Can you work these out from the model? Positions are in its coordinate system, mm. A direction names the side the tool comes from. Give positions to 0.01 mm unless a question says otherwise; leave off trailing zeros. Loops run counter-clockwise (first coordinate to the right, second up) from the corner with the lowest first, then second, coordinate; pieces in that order, holes last. Notation, with made-up numbers: (31, 59) - (74, 59) arc R22 cw to (74, 87) - close; hole circle Ø9 at (12, 85.25). An arc over 180 degrees is marked (long way). Answer as a JSON object with one key per item and string values. Group by question number.
Item 1: Thinking about a two-plate mould opening in X: for faces 3 (the flat face through (0, -2, 3)), 4 (the cylindrical face through (6.302, -1.973, 4.177)), 5 (the flat face through (3.8, 0, 3.1)), 6 (the flat face through (10, -2, 1)), which applies, pulls with the +X half, pulls with the -X half, needs draft (parallel to the pull), parting line crosses it, or undercut?
Item 2: Suppose I cut it at A-A on z = 1.25. Write out the boundary of the cut face in (x, y).
Item 3: Will this pin go through, and if not, where does the flat tip stop? pin 1 (1 mm diameter, centred on x = 5.5, y = -0.5, fed in from -Z).
Item 4: Which directions (+Z, -Z, +X, -X, +Y, -Y) give clear straight access to the entire face, cutting with the end or side of a thin tool? Please do faces 1 (the flat face through (9, -2, 1)), 2 (the flat face through (9.4, -2, 0)).
Item 5: Please list where these lines run through material, in increasing order: L1, parallel to Y at x = 2, z = 2.7; L2, parallel to X at y = -3.75, z = 2.8; L3, parallel to X at y = -3.55, z = 3.3.
Item 6: Suppose I cut it at B-B on x = 2. Write out the boundary of the cut face in (y, z), and give its area (3 significant figures).
from build123d import *

# Parameters (mm, degrees)
F1_DEPTH = 4
F3_R     = 0.1
F2_R     = 0.75
F4_DEPTH = 25


# Not quite as in the source:
# - ends of sketch curves that miss each other by under 0.0002 mm in the source are joined


with BuildPart() as f1:
    # F0 (on Front) → F1 (new body)
    with BuildSketch(Plane.XZ):
        with BuildLine():
            Line((0, 5), (0, 0))
            Line((0, 0), (3.7373243831, 0))
            Line((3.7373243831, 0), (3.7373243831, 1.5373318456))
            ThreePointArc((3.7373243831, 1.5373318456), (6.3598005329, 4.1775164411), (8.9999850781, 1.5550552132))
            Line((8.9999850781, 1.5550552132), (9, 1.5461935545))
            Line((9, 1.5461935545), (9, 0))
            Line((9, 0), (9.6543736474, 0))
            ThreePointArc((9.6543736474, 0), (9.9125401886, 0.7540174245), (10, 1.5461935545))
            ThreePointArc((10, 1.5461935545), (9.3062869056, 3.680900869), (7.4901947663, 5))
            Line((7.4901947663, 5), (5.2471296168, 5))
            Line((5.2471296168, 5), (0, 5))
        make_face()
        with BuildLine():
            Line((10, 0), (10, 1.5461935545))
            ThreePointArc((10, 1.5461935545), (9.9125401886, 0.7540174245), (9.6543736474, 0))
            Line((9.6543736474, 0), (10, 0))
        make_face()
    extrude(amount=F1_DEPTH)

    # F3
    f3_edges = [f1.edges().sort_by_distance(p)[0] for p in [
        (3.745097, -4, 5),
        (0, -2, 5),
        (0, -4, 2.5),
        (6.359793, -4, 4.177516),
        (3.737324, -2, 0),
        (1.868662, -4, 0),
        (9.5, -4, 0),
        (10, -2, 0),
        (9.5, 0, 0),
        (10, 0, 0.773097),
        (10, -4, 0.773097),
        (3.737324, 0, 0.768666),
        (3.745097, 0, 5),
        (0, 0, 2.5),
        (1.868662, 0, 0),
        (0, -2, 0),
    ]]
    fillet(f3_edges, radius=F3_R)

    # F2 (on face) → F4 (cut)
    with BuildSketch(Plane.XY.offset(5)):
        with Locations((2, -2)):
            Circle(F2_R)
    extrude(amount=-F4_DEPTH, mode=Mode.SUBTRACT)


solid = f1.part
Worked out:
{
 "1": {"face 3": "pulls with the -X half", "face 4": "undercut", "face 5": "needs draft", "face 6": "pulls with the +X half"},
 "2": {"outline": "(0, -3.9) arc R0.1 ccw to (0.1, -4) - (3.64, -4) arc R0.1 ccw to (3.74, -3.9) - (3.74, -0.1) arc R0.1 ccw to (3.64, 0) - (0.1, 0) arc R0.1 ccw to (0, -0.1) - close; (9, -3.9) arc R0.1 ccw to (9.1, -4) - (9.9, -4) arc R0.1 ccw to (10, -3.9) - (10, -0.1) arc R0.1 ccw to (9.9, 0) - (9.1, 0) arc R0.1 ccw to (9, -0.1) - close; hole circle Ø1.5 at (2, -2)"},
 "3": {"pin 1": "stops at z = 3.79"},
 "4": {"face 1": "-Z, +Y, -Y", "face 2": "-Z, +X, -X, +Y, -Y"},
 "5": {"L1": "y = -4 to -2.75, -1.25 to 0", "L2": "x = 0 to 4.06, 8.68 to 9.78", "L3": "x = 0 to 4.41, 8.33 to 9.55"},
 "6": {"outline": "(-4, 0.1) arc R0.1 ccw to (-3.9, 0) - (-2.75, 0) - (-2.75, 5) - (-3.9, 5) arc R0.1 ccw to (-4, 4.9) - close; (-1.25, 0) - (-0.1, 0) arc R0.1 ccw to (0, 0.1) - (0, 4.9) arc R0.1 ccw to (-0.1, 5) - (-1.25, 5) - close", "area": "12.5 mm2"}
}
